For this review, take the finished solid that the model builds, in its own axes (mm). A direction names the side the tool comes from. Give positions to 0.01 mm unless a question says otherwise; leave off trailing zeros. Write each loop counter-clockwise with the first axis right and the second up, starting at its lowest first coordinate (ties: lowest second). Pieces come first, ordered by that corner, then holes. Notation, with made-up numbers: M 82.5,22.25 L 101.5,22.25 A9 cw 101.5,26.25 Z; hole C 12,80.25 d8. An arc over 180 degrees is marked long. Use one line per item in the form item = value. Start each with the question number.
Q1. Consider section C-C on y = 27.5. Write out the cut boundary in (x, z), and give its area (3 significant figures).
Q2. Consider section B-B on x = 0. Write out the cut boundary in (y, z), and give its area (3 significant figures).
Q3. Consider section A-A on z = 0. Write out the cut boundary in (x, y).
Q4. Tool access review of faces 4 (the cylindrical face through (-1.802, 25.53, -5.723)), 5 (the flat face through (0, -6.274, 0)), 6 (the cylindrical face through (-0.66, 7.247, 14.985)): name each direction out of +Z, -Z, +X, -X, +Y, -Y from which nothing blocks a thin tool from reaching the whole face with its end or side.
Q5. Mouldability with a two-part tool opening along Z and no side actions: class faces 1 (the flat face through (-4.5, 11.726, -4.5)), 2 (the cylindrical face through (4.88, 1.63, 1.08)), 3 (the cylindrical face through (11.56, 8.68, 15.08)) as released by +Z, released by -Z, zero draft, split by the parting line, or undercut.
Q6. Consider section D-D on z = -7. Write out the cut boundary in (x, y).
Q7. Clearance check with flat-ended pins moving along their axes: pin 1 Ø1.5 at (y, z) = (17.5, 3) entering from +X; pin 2 Ø5 at (y, z) = (33.5, -2) entering from -X; pin 3 Ø4 at (x, z) = (9, 2) entering from -Y. State where each tip first meets the part, or that it passes through.
Q8. For probe 1 along X at (y, z) = (7, 0); probe 2 along X at (y, z) = (6, 2); probe 3 along Y at (x, z) = (11.5, -12.5), list the stretches that pass through material, from the lowest coordinate up. Write a range as [from, to].
```python
from build123d import *

# Parameters (mm, degrees)
CHAMFER1_SIZE = 1
CHAMFER2_SIZE = 2


with BuildPart() as part:
    # Sketch1 → Revolve1 (revolve)
    with BuildSketch(Plane.XY, mode=Mode.PRIVATE) as revolve1_sk:
        Polygon((0, 41.725973007), (-6, 41.725973007), (-6, 11.725973007), (-19, 11.725973007), (-19, 5.725973007), (-15, 5.725973007), (-15, 8.725973007), (-5, 8.725973007), (-5, -6.274026993), (0, -6.274026993), align=None)
    revolve(revolve1_sk.sketch.rotate(Axis((0, 0, 0), (0, 1, 0)), 270), axis=Axis((0, 0, 0), (0, 1, 0)))

    # Chamfer1
    chamfer1_edges = [part.edges().sort_by_distance(p)[0] for p in [
        (0, -6.274026993, 5),
    ]]
    chamfer(chamfer1_edges, length=CHAMFER1_SIZE)

    # Chamfer2
    chamfer2_edges = [part.edges().sort_by_distance(p)[0] for p in [
        (0, 41.725973007, 6),
    ]]
    chamfer(chamfer2_edges, length=CHAMFER2_SIZE)


solid = part.part
```
Working result:
q1.outline = C 0,0 d12
q1.area = 113 mm²
q2.outline = M -6.27,-4 L -5.27,-5 L 8.73,-5 L 8.73,-15 L 5.73,-15 L 5.73,-19 L 11.73,-19 L 11.73,-6 L 39.73,-6 L 41.73,-4 L 41.73,4 L 39.73,6 L 11.73,6 L 11.73,19 L 5.73,19 L 5.73,15 L 8.73,15 L 8.73,5 L -5.27,5 L -6.27,4 Z
q2.area = 643 mm²
q3.outline = M -19,5.73 L -15,5.73 L -15,8.73 L -5,8.73 L -5,-5.27 L -4,-6.27 L 4,-6.27 L 5,-5.27 L 5,8.73 L 15,8.73 L 15,5.73 L 19,5.73 L 19,11.73 L 6,11.73 L 6,39.73 L 4,41.73 L -4,41.73 L -6,39.73 L -6,11.73 L -19,11.73 Z
q4.face_4 = +Y
q4.face_5 = +Z, -Z, +X, -X, -Y
q4.face_6 = -Y
q5.face_1 = zero draft
q5.face_2 = undercut
q5.face_3 = split by the parting line
q6.outline = M -17.66,5.73 L -13.27,5.73 L -13.27,8.73 L 13.27,8.73 L 13.27,5.73 L 17.66,5.73 L 17.66,11.73 L -17.66,11.73 Z
q7.pin_1 = 5.56
q7.pin_2 = -6
q7.pin_3 = 8.73
q8.probe_1 = [-19, -15], [-5, 5], [15, 19]
q8.probe_2 = [-18.89, -14.87], [-4.58, 4.58], [14.87, 18.89]
q8.probe_3 = [5.73, 11.73]
